from build123d import *

# Parameters (mm, degrees)
SKETCH1_R               = 34.5
SKETCH1_R_2             = 4
BOSS_EXTRUDE1_DEPTH     = 4.5
SKETCH2_W               = 1.5
SKETCH2_H               = 2.65
CUT_EXTRUDE1_DEPTH      = 49.997448913
CUT_EXTRUDE1_DEPTH_BACK = 49.997448913
SKETCH4_W               = 1.55
SKETCH4_H               = 1.5


with BuildPart() as part:
    # Sketch1 → Boss-Extrude1 (new body)
    with BuildSketch(Plane.XY):
        Circle(SKETCH1_R)
        with Locations((5.75, 5.75)):
            Circle(SKETCH1_R_2, mode=Mode.SUBTRACT)
        with Locations((8.338190451, 15.409258263)):
            Circle(SKETCH1_R_2, mode=Mode.SUBTRACT)
        with Locations((17.997448714, 17.997448714)):
            Circle(SKETCH1_R_2, mode=Mode.SUBTRACT)
        with Locations((15.409258263, 8.338190451)):
            Circle(SKETCH1_R_2, mode=Mode.SUBTRACT)
        with Locations((25.068516526, 5.75)):
            Circle(SKETCH1_R_2, mode=Mode.SUBTRACT)
        with Locations((5.75, 25.068516526)):
            Circle(SKETCH1_R_2, mode=Mode.SUBTRACT)
        with Locations((25.068556101, -5.749960425)):
            Circle(SKETCH1_R_2, mode=Mode.SUBTRACT)
        with Locations((15.409297838, -8.338150876)):
            Circle(SKETCH1_R_2, mode=Mode.SUBTRACT)
        with Locations((17.997488289, -17.997409139)):
            Circle(SKETCH1_R_2, mode=Mode.SUBTRACT)
        with Locations((8.338230026, -15.409218688)):
            Circle(SKETCH1_R_2, mode=Mode.SUBTRACT)
        with Locations((5.750039575, -25.068476951)):
            Circle(SKETCH1_R_2, mode=Mode.SUBTRACT)
        with Locations((5.750039575, -5.749960425)):
            Circle(SKETCH1_R_2, mode=Mode.SUBTRACT)
        with Locations((-5.74992085, -25.068516526)):
            Circle(SKETCH1_R_2, mode=Mode.SUBTRACT)
        with Locations((-8.338111301, -15.409258263)):
            Circle(SKETCH1_R_2, mode=Mode.SUBTRACT)
        with Locations((-17.997369564, -17.997448714)):
            Circle(SKETCH1_R_2, mode=Mode.SUBTRACT)
        with Locations((-15.409179113, -8.338190451)):
            Circle(SKETCH1_R_2, mode=Mode.SUBTRACT)
        with Locations((-25.068437376, -5.75)):
            Circle(SKETCH1_R_2, mode=Mode.SUBTRACT)
        with Locations((-5.74992085, -5.75)):
            Circle(SKETCH1_R_2, mode=Mode.SUBTRACT)
        with Locations((-25.068476951, 5.749960425)):
            Circle(SKETCH1_R_2, mode=Mode.SUBTRACT)
        with Locations((-15.409218688, 8.338150876)):
            Circle(SKETCH1_R_2, mode=Mode.SUBTRACT)
        with Locations((-17.997409139, 17.997409139)):
            Circle(SKETCH1_R_2, mode=Mode.SUBTRACT)
        with Locations((-8.338150876, 15.409218688)):
            Circle(SKETCH1_R_2, mode=Mode.SUBTRACT)
        with Locations((-5.749960425, 25.068476951)):
            Circle(SKETCH1_R_2, mode=Mode.SUBTRACT)
        with Locations((-5.749960425, 5.749960425)):
            Circle(SKETCH1_R_2, mode=Mode.SUBTRACT)
    extrude(amount=BOSS_EXTRUDE1_DEPTH)

    # Sketch2 → Cut-Revolve1 (revolve, cut)
    with BuildSketch(Plane(origin=(0, 0, 0), x_dir=(0, 0, -1), z_dir=(1, 0, 0))):
        with Locations((-0.75, 33.175)):
            Rectangle(SKETCH2_W, SKETCH2_H)
        with Locations((-3.75, 33.175)):
            Rectangle(SKETCH2_W, SKETCH2_H)
    revolve(axis=Axis((0, 0, 0), (0, 0, 1)), mode=Mode.SUBTRACT)

    # Sketch4 → Cut-Extrude1 (cut, two sides: drawn at the far end of the back side and taken through both)
    with BuildSketch(Plane(origin=(0, 0, 0), x_dir=(1, 0, 0), z_dir=(0, 1, 0)).offset(-CUT_EXTRUDE1_DEPTH_BACK)):
        with Locations((0, -0.75)):
            Rectangle(SKETCH4_W, SKETCH4_H)
    extrude(amount=CUT_EXTRUDE1_DEPTH + CUT_EXTRUDE1_DEPTH_BACK, mode=Mode.SUBTRACT)


solid = part.part
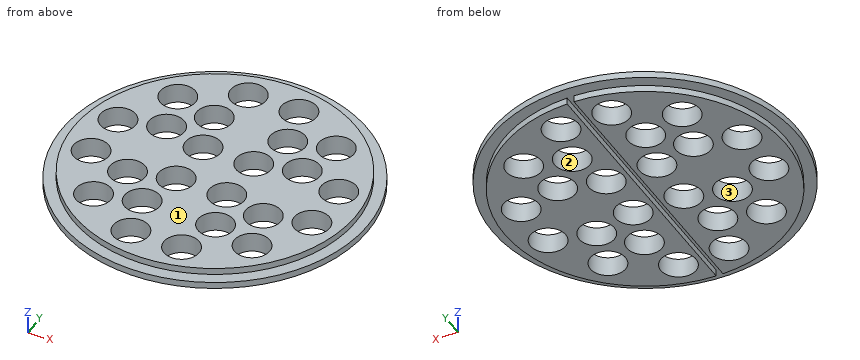
Model file for the job. Use its own axes, mm. Face numbers are marked on the shaded views. Give positions to 0.01 mm unless a question says otherwise; leave off trailing zeros. Loops run counter-clockwise (first coordinate to the right, second up) from the corner with the lowest first, then second, coordinate; pieces in that order, holes last.
1) Flat gauge pins, fed straight in: pin 1 Ø1.6 at (y, z) = (13, 1) entering from +X; pin 2 Ø1 at (y, z) = (-6, 3) entering from -X; pin 3 Ø1.2 at (y, z) = (4, 0.5) entering from -X. Where does each tip first touch, or does it go through?
2) Pull direction Y, two halves, no side cores. Call the marked faces 1, 2 and 3: +Y half, -Y half, draft (parallel to the pull), parting line (faces both ways), or undercut.
3) Wall check: line 1 (X direction, y = -12, z = 0.3) (3 decimals); line 2 (X direction, y = -2.5, z = 1.65); line 3 (Y direction, x = -17, z = 0.55). Give the ranges that are in metal, low to high.
4) Saw through at A-A (y = 0). Write the cut outline in (x, z) (3 decimals).
5) Saw through at B-B (z = 2.3). Count the separate pieces of the cut face and the enclosed holes in it, plus the area to 3 significant figures.
Answer block:
1. pin 1: stops at x = 32.2
1. pin 2: stops at x = -34.06
1. pin 3: stops at x = -31.67
2. face 1: draft
2. face 2: undercut
2. face 3: undercut
3. line 1: x = -29.503 to -17.019, -13.799 to -10.43, -6.246 to -0.775, 0.775 to 6.246, 10.43 to 13.8, 17.019 to 29.503
3. line 2: x = -34.41 to -27.4, -22.74 to -8.08, -3.42 to 3.42, 8.08 to 22.74, 27.4 to 34.41
3. line 3: y = -26.93 to -21.87, -14.12 to -12.01, -4.67 to 4.67, 12.01 to 14.12, 21.87 to 26.93
4. outline: (-34.5, 1.5) - (-31.85, 1.5) - (-31.85, 0) - (-0.775, 0) - (-0.775, 1.5) - (0.775, 1.5) - (0.775, 0) - (31.85, 0) - (31.85, 1.5) - (34.5, 1.5) - (34.5, 3) - (31.85, 3) - (31.85, 4.5) - (-31.85, 4.5) - (-31.85, 3) - (-34.5, 3) - close
5. separate pieces: 1
5. enclosed holes: 24
5. area: 2,530 mm2
